Source: CAD feature listing. Evaluate the final solid. Frame: model axes, mm. A direction names the side the tool comes from. Coordinates: 2 decimals unless noted, no trailing zeros. Loops run counter-clockwise (first coordinate to the right, second up) from the corner with the lowest first, then second, coordinate; pieces in that order, holes last.
Item 1: Line query: probe 1 along Z at (x, y) = (-20, 0) (3 decimals); probe 2 along Y at (x, z) = (-23, 12.7) (3 decimals); probe 3 along Z at (x, y) = (-19.5, 9.5). Output: solid intervals per line, ascending.
Item 2: Section query B-B, the plane x = -23. Return the cut outline in (y, z) (3 decimals).
Item 3: Reachability of faces 5 (the cylindrical face through (-9.617, 0.023, 1.905)), 6 (the cylindrical face through (-12.159, 1.491, 23.495)), 7 (the cylindrical face through (-30.089, 11.172, 23.951)), 8 (the cylindrical face through (-29.693, -11.172, 23.951)) from +Z, -Z, +X, -X, +Y, -Y: full face, straight path, thin tool, end or side. Return the list, or none.
Item 4: Pull-direction query (Y, two-part tool) for faces 1 (the flat face through (-17, 0, 0)), 2 (the cylindrical face through (7.8, 10.62, 23.87)), 3 (the flat face through (14.663, -22.792, 12.522)), 4 (the cylindrical face through (7.534, -10.321, 1.449)); classes: +Y half, -Y half, draft (parallel to the pull), parting line (faces both ways), or undercut.
Item 5: Pin query (flat end, axial travel): pin 1 Ø1.5 at (x, z) = (-25.5, 5) entering from +Y; pin 2 Ø5 at (x, z) = (-17, 22) entering from +Y; pin 3 Ø12 at (x, z) = (-29.5, 10.5) entering from -Y. Return the tip coordinate at first contact, or that it passes through.
Item 6: Section query C-C, the plane z = 12.7. Return the cut outline in (x, y) (3 decimals), then the cut area to 3 significant figures.
Item 7: Section query A-A, the plane z = 22.25. Return the cut outline in (x, y), then the cut area to 3 significant figures.
```python
from build123d import *

# Parameters (mm, degrees)
F1_DEPTH = 25.4
F4_R     = 10.795
F5_DEPTH = 35.56
F3_R     = 10.795
F6_DEPTH = 35.56
F2_R     = 10.795
F7_DEPTH = 35.56
F8_R     = 5.08


with BuildPart() as f1:
    # F0 (on Top) → F1 (new body)
    with BuildSketch(Plane.XY):
        Polygon((16.03946, 21.997045), (-5.957585, 34.697045), (-18.657585, 12.7), (-44.057585, 12.7), (-44.057585, -12.7), (-18.657585, -12.7), (-5.957585, -34.697045), (16.03946, -21.997045), (3.33946, 0), align=None)
    extrude(amount=F1_DEPTH)

    # F4 (on face) → F5 (cut)
    with BuildSketch(Plane(origin=(-44.057585, 0, 0), x_dir=(0, -1, 0), z_dir=(-1, 0, 0))):
        with Locations((0, 12.7)):
            Circle(F4_R)
    extrude(amount=-F5_DEPTH, mode=Mode.SUBTRACT)

    # F3 (on face) → F6 (cut)
    with BuildSketch(Plane(origin=(13.534865, 23.443074, 0), x_dir=(-0.866025, 0.5, 0), z_dir=(0.5, 0.866025, 0))):
        with Locations((9.807943, 12.7)):
            Circle(F3_R)
    extrude(amount=-F6_DEPTH, mode=Mode.SUBTRACT)

    # F2 (on face) → F7 (cut)
    with BuildSketch(Plane(origin=(13.534865, -23.443074, 0), x_dir=(0.866025, 0.5, 0), z_dir=(0.5, -0.866025, 0))):
        with Locations((-9.807943, 12.7)):
            Circle(F2_R)
    extrude(amount=-F7_DEPTH, mode=Mode.SUBTRACT)

    # F8
    f8_edges = [f1.edges().sort_by_distance(p)[0] for p in [
        (-31.357585, -12.7, 25.4),
        (-12.307585, -23.698523, 25.4),
        (-31.357585, 12.7, 25.4),
        (-12.307585, 23.698523, 25.4),
        (9.68946, 10.998523, 25.4),
        (9.68946, -10.998523, 25.4),
        (-31.357585, -12.7, 0),
        (-12.307585, -23.698523, 0),
        (9.68946, -10.998523, 0),
        (9.68946, 10.998523, 0),
        (-31.357585, 12.7, 0),
        (-12.307585, 23.698523, 0),
    ]]
    fillet(f8_edges, radius=F8_R)


solid = f1.part
```
Verdict:
1. probe 1: z = 0 to 1.905, 23.495 to 25.4
1. probe 2: y = -12.7 to -10.795, 10.795 to 12.7
1. probe 3: z = 0.36 to 7.57, 17.83 to 25.04
2. outline: (-12.7, 5.08) arc R5.08 ccw to (-7.62, 0) - (7.62, 0) arc R5.08 ccw to (12.7, 5.08) - (12.7, 20.32) arc R5.08 ccw to (7.62, 25.4) - (-7.62, 25.4) arc R5.08 ccw to (-12.7, 20.32) - close; hole circle Ø21.59 at (0, 12.7)
3. face 5: -X
3. face 6: none
3. face 7: +Z, -X, +Y
3. face 8: +Z, -X, -Y
4. face 1: draft
4. face 2: undercut
4. face 3: -Y half
4. face 4: undercut
5. pin 1: stops at y = 12.7
5. pin 2: stops at y = 19.54
5. pin 3: stops at y = -12.7
6. outline: (-44.058, -12.7) - (-18.658, -12.7) - (-5.958, -34.697) - (-4.308, -33.745) - (-17.558, -10.795) - (-44.058, -10.795) - close; (-44.058, 10.795) - (-17.558, 10.795) - (-4.308, 33.745) - (-5.958, 34.697) - (-18.658, 12.7) - (-44.058, 12.7) - close; (1.14, 0) - (14.39, -22.95) - (16.039, -21.997) - (3.339, 0) - (16.039, 21.997) - (14.39, 22.95) - close
6. area: 297 mm2
7. outline: (-44.06, -12.32) - (-18.44, -12.32) - (-5.63, -34.51) - (0.68, -30.86) - (-14.23, -5.03) - (-44.06, -5.03) - close; (-44.06, 5.03) - (-14.23, 5.03) - (0.68, 30.86) - (-5.63, 34.51) - (-18.44, 12.32) - (-44.06, 12.32) - close; (-5.51, 0) - (9.4, -25.83) - (15.71, -22.19) - (2.9, 0) - (15.71, 22.19) - (9.4, 25.83) - close
7. area: 1,210 mm2
